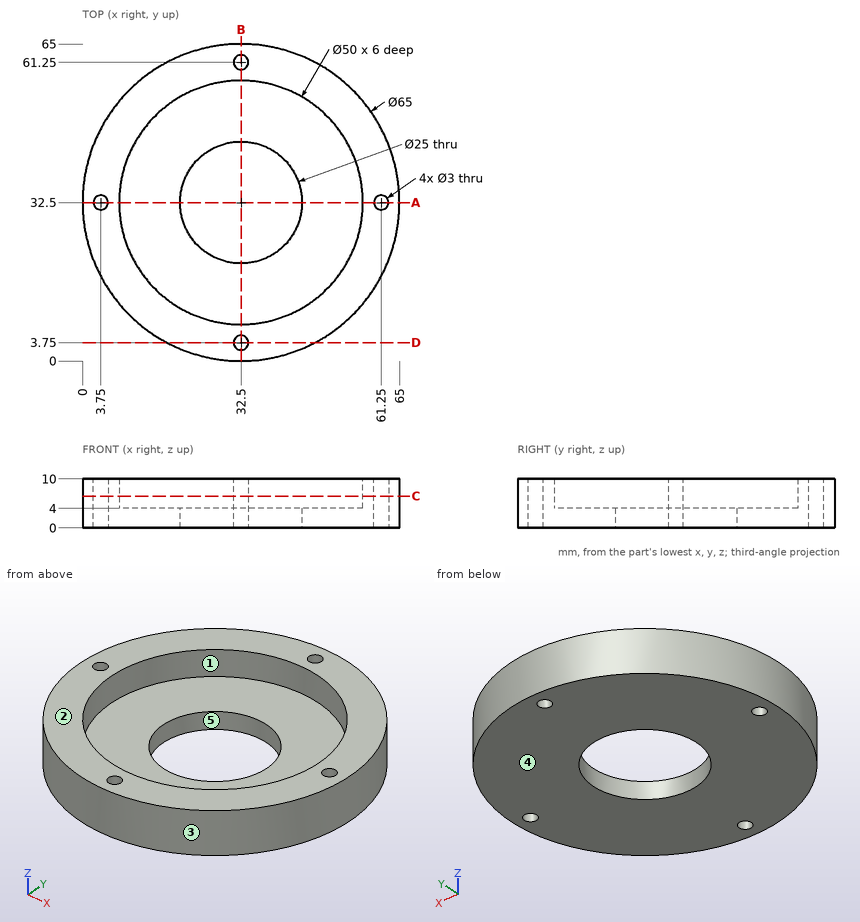
Can you work these out from the drawing? Everything is in mm from the part's minimum corner. A direction names the side the tool comes from. Coordinates: 2 decimals unless noted, no trailing zeros. Loops run counter-clockwise (first coordinate to the right, second up) from the corner with the lowest first, then second, coordinate; pieces in that order, holes last.
1. Imagine slicing it at D-D, the plane y = 3.75. Please give me the cut outline in (x, z), and give its area (3 significant figures).
2. I need wall thicknesses on L1, parallel to Y at x = 32.5, z = 7.05; L2, parallel to Y at x = 32.5, z = 1; L3, parallel to Z at x = 14.5, y = 29.5. Which ranges of each line are inside material? Lowest first, please.
3. Imagine slicing it at C-C, the plane z = 6.5. Please give me the cut outline in (x, y).
4. For the marked faces 1 and 2, which set-ups out of +Z, -Z, +X, -X, +Y, -Y let a thin tool reach every point of the face, with its end or its side?
5. If we mould it in two halves opening along X, with no side actions, what happens to the marked faces 3, 4 and 5? For each: pulls with the +X half, pulls with the -X half, needs draft (parallel to the pull), parting line crosses it, or undercut.
6. Imagine slicing it at A-A, the plane y = 32.5. Please give me the cut outline in (x, z).
7. For P1, Ø4, axis at x = 58.5, z = 8.5, coming from the +Y side; P2, Ø25, axis at x = 43, y = 38, coming from the +Z side; P3, Ø5, axis at x = 29.5, z = 7, coming from the -Y side, each with a flat end and sliding along its axis, tell me the tip position at first contact or that it passes through.
Taken from the geometry:
1. outline: (17.34, 0) - (31, 0) - (31, 10) - (17.34, 10) - close; (34, 0) - (47.66, 0) - (47.66, 10) - (34, 10) - close
1. area: 273 mm2
2. L1: y = 0 to 2.25, 5.25 to 7.5, 57.5 to 59.75, 62.75 to 65
2. L2: y = 0 to 2.25, 5.25 to 20, 45 to 59.75, 62.75 to 65
2. L3: z = 0 to 4
3. outline: circle Ø65 at (32.5, 32.5); hole circle Ø3 at (3.75, 32.5); hole circle Ø50 at (32.5, 32.5); hole circle Ø3 at (32.5, 3.75); hole circle Ø3 at (32.5, 61.25); hole circle Ø3 at (61.25, 32.5)
4. face 1: +Z
4. face 2: +Z, +X, -X, +Y, -Y
5. face 3: parting line crosses it
5. face 4: needs draft
5. face 5: undercut
6. outline: (0, 0) - (2.25, 0) - (2.25, 10) - (0, 10) - close; (5.25, 0) - (20, 0) - (20, 4) - (7.5, 4) - (7.5, 10) - (5.25, 10) - close; (45, 0) - (59.75, 0) - (59.75, 10) - (57.5, 10) - (57.5, 4) - (45, 4) - close; (62.75, 0) - (65, 0) - (65, 10) - (62.75, 10) - close
7. P1: stops at y = 54.41
7. P2: stops at z = 4
7. P3: stops at y = 0
